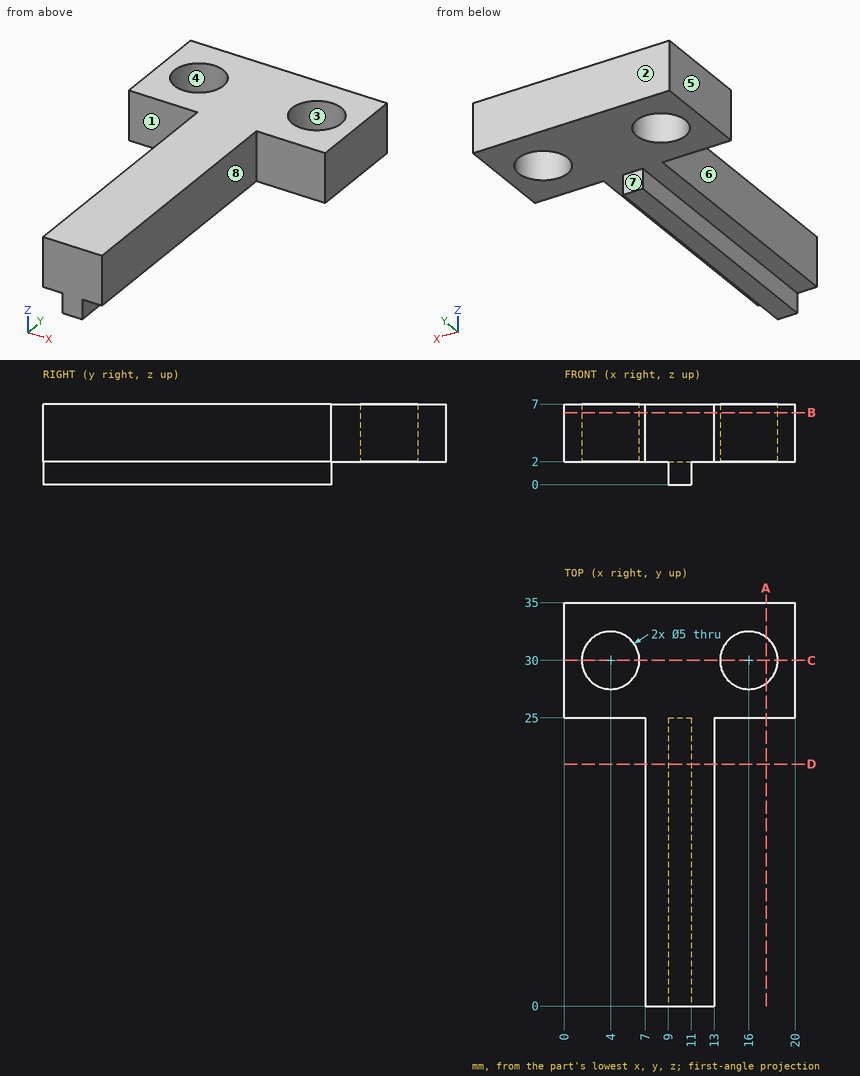
Design review of the part shown in the three views and the two pictorial views. Dimensions are in mm from the part's minimum x, y and z. A direction names the side the tool comes from. Round coordinates to 2 decimals unless told otherwise and drop trailing zeros. Write each loop counter-clockwise with the first axis right and the second up, starting at its lowest first coordinate (ties: lowest second). Pieces come first, ordered by that corner, then holes. Notation, with made-up numbers: (-34, 86.25) -> (11, 86.25) arc R6 ccw to (11, 91.25) -> close; hole circle Ø9 at (-38.5, 84.5). An arc over 180 degrees is marked (long way). One line per question, with ' | ' between items. Start each with the question number.
1) Mouldability with a two-part tool opening along Y and no side actions: class the marked faces 1, 2, 3 and 4 as +Y half, -Y half, draft (parallel to the pull), parting line (faces both ways), or undercut.
2) Add section B-B (z = 6.25). Write out the cut boundary in (x, y), and give its area (3 significant figures).
3) Add section C-C (y = 30). Write out the cut boundary in (x, z).
4) For pin 1 Ø1 at (y, z) = (20, 6) entering from +X; pin 2 Ø0.6 at (y, z) = (18.5, 1) entering from +X; pin 3 Ø2.5 at (x, z) = (17.5, 5) entering from -Y, all flat-tipped, find the tip position at first contact; note any pin that passes through.
5) Machinability: for the marked faces 5, 6, 7 and 8, which of the approach directions +Z, -Z, +X, -X, +Y, -Y give a long, thin tool a straight path to every point of the face, cutting with its end or side? Answer none if there is none.
6) Add section A-A (x = 17.5). Write out the cut boundary in (y, z).
7) Add section D-D (y = 21). Write out the cut boundary in (x, z), and give its area (3 significant figures).
8) Wall thickness on line 1 along X through (y, z) = (29.5, 2.75); line 2 along Y through (x, z) = (16, 4.45); line 3 along X through (y, z) = (2.5, 6): over which ranges is each line inside the solid? List them lowest first.
Reported:
1) face 1: -Y half | face 2: +Y half | face 3: undercut | face 4: undercut
2) outline: (0, 25) -> (7, 25) -> (7, 0) -> (13, 0) -> (13, 25) -> (20, 25) -> (20, 35) -> (0, 35) -> close; hole circle Ø5 at (4, 30); hole circle Ø5 at (16, 30) | area: 311 mm²
3) outline: (0, 2) -> (1.5, 2) -> (1.5, 7) -> (0, 7) -> close; (6.5, 2) -> (13.5, 2) -> (13.5, 7) -> (6.5, 7) -> close; (18.5, 2) -> (20, 2) -> (20, 7) -> (18.5, 7) -> close
4) pin 1: stops at x = 13 | pin 2: stops at x = 11 | pin 3: stops at y = 25
5) face 5: +Z, -Z, -X, +Y, -Y | face 6: +Z, -Z, -X, -Y | face 7: -Z, +X, -X, +Y | face 8: +Z, -Z, +X, -Y
6) outline: (25, 2) -> (28, 2) -> (28, 7) -> (25, 7) -> close; (32, 2) -> (35, 2) -> (35, 7) -> (32, 7) -> close
7) outline: (7, 2) -> (9, 2) -> (9, 0) -> (11, 0) -> (11, 2) -> (13, 2) -> (13, 7) -> (7, 7) -> close | area: 34.0 mm²
8) line 1: x = 0 to 1.55, 6.45 to 13.55, 18.45 to 20 | line 2: y = 25 to 27.5, 32.5 to 35 | line 3: x = 7 to 13
